Part model, mm, in its own coordinate system. A direction names the side the tool comes from. Coordinates: 2 decimals unless noted, no trailing zeros. Loops run counter-clockwise (first coordinate to the right, second up) from the corner with the lowest first, then second, coordinate; pieces in that order, holes last. Notation, with made-up numbers: (-16.5, -2.5) - (30.5, -2.5) arc R26 cw to (30.5, 17.5) - close; hole circle Ø7 at (-20.5, 66.5). An arc over 180 degrees is marked (long way). Use a Markdown table: item, result. Add a question column.
1) Band-saw the part on C-C (x = 13.5). Give the cut face in (y, z), plus the area to 3 significant figures.
2) Band-saw the part on D-D (z = 18.5). Give the cut face in (x, y).
3) Tool access for faces 5 (the face through (1.5, -2, 30)), 6 (the face through (5.301, -2.465, 5.285)), 7 (the face through (20, -2, -1.5)): list every direction of +Z, -Z, +X, -X, +Y, -Y with a clear straight run to the whole face (end or side of a thin tool).
4) Band-saw the part on B-B (y = -1.7). Give the cut face in (x, z), plus the area to 3 significant figures.
5) Pull direction X, two halves, no side cores. Call faces 1 (the face through (14, -2, 5)), 2 (the face through (-0.54, -2.46, -2.44)), 3 (the face through (-5, -2, 16)), 4 (the face through (4.715, -2.465, 32.699)): +X half, -X half, draft (parallel to the pull), parting line (faces both ways), or undercut.
6) Probe probe 1 along Z at (x, y) = (0, -2.6); probe 2 along X at (y, z) = (-1.5, 27). List the from-to ranges inside material, lowest first. Write a range as [from, to].
7) Band-saw the part on A-A (z = 27.5). Give the cut face in (x, y), plus the area to 3 significant figures.
8) Drop flat-ended pins along their axis: P1, Ø1.5, axis at x = 0.5, z = 27.5, coming from the +Y side; P2, Ø2.5, axis at y = -3, z = 22.5, coming from the +X side. Give the stop position or say it passes through.
from build123d import *

# Parameters (mm, degrees)
F0_R     = 2.5
F1_DEPTH = 5


with BuildPart() as f1:
    # F0 (on Front) → F1 (new body)
    with BuildSketch(Plane.XZ):
        with BuildLine():
            Line((-2.5, 33), (-4, 33))
            ThreePointArc((-4, 33), (-4.707107, 32.707107), (-5, 32))
            Line((-5, 32), (-5, 0))
            ThreePointArc((-5, 0), (-3.535534, -3.535534), (0, -5))
            Line((0, -5), (22.5, -5))
            ThreePointArc((22.5, -5), (23.207107, -4.707107), (23.5, -4))
            Line((23.5, -4), (23.5, -2.5))
            ThreePointArc((23.5, -2.5), (23.207107, -1.792893), (22.5, -1.5))
            Line((22.5, -1.5), (17.5, -1.5))
            ThreePointArc((17.5, -1.5), (16, 0), (17.5, 1.5))
            Line((17.5, 1.5), (22.5, 1.5))
            ThreePointArc((22.5, 1.5), (23.207107, 1.792893), (23.5, 2.5))
            Line((23.5, 2.5), (23.5, 4))
            ThreePointArc((23.5, 4), (23.207107, 4.707107), (22.5, 5))
            Line((22.5, 5), (6, 5))
            ThreePointArc((6, 5), (5.292893, 5.292893), (5, 6))
            Line((5, 6), (5, 32))
            ThreePointArc((5, 32), (4.707107, 32.707107), (4, 33))
            Line((4, 33), (2.5, 33))
            ThreePointArc((2.5, 33), (1.792893, 32.707107), (1.5, 32))
            Line((1.5, 32), (1.5, 27))
            ThreePointArc((1.5, 27), (0, 25.5), (-1.5, 27))
            Line((-1.5, 27), (-1.5, 32))
            ThreePointArc((-1.5, 32), (-1.792893, 32.707107), (-2.5, 33))
        make_face()
        Circle(F0_R, mode=Mode.SUBTRACT)
    extrude(amount=F1_DEPTH)


solid = f1.part
Answer block:
| question | item | result |
|---|---|---|
| 1 | outline | (-5, -5) - (0, -5) - (0, 5) - (-5, 5) - close |
| 1 | area | 50.0 mm2 |
| 2 | outline | (-5, -5) - (5, -5) - (5, 0) - (-5, 0) - close |
| 3 | face 5 | +Z, +Y, -Y |
| 3 | face 6 | +Z, +X, +Y, -Y |
| 3 | face 7 | +X, +Y, -Y |
| 4 | outline | (-5, 0) arc R5 ccw to (0, -5) - (22.5, -5) arc R1 ccw to (23.5, -4) - (23.5, -2.5) arc R1 ccw to (22.5, -1.5) - (17.5, -1.5) arc R1.5 cw to (17.5, 1.5) - (22.5, 1.5) arc R1 ccw to (23.5, 2.5) - (23.5, 4) arc R1 ccw to (22.5, 5) - (6, 5) arc R1 cw to (5, 6) - (5, 32) arc R1 ccw to (4, 33) - (2.5, 33) arc R1 ccw to (1.5, 32) - (1.5, 27) arc R1.5 cw to (-1.5, 27) - (-1.5, 32) arc R1 ccw to (-2.5, 33) - (-4, 33) arc R1 ccw to (-5, 32) - close; hole circle Ø5 at (0, 0) |
| 4 | area | 495 mm2 |
| 5 | face 1 | draft |
| 5 | face 2 | undercut |
| 5 | face 3 | -X half |
| 5 | face 4 | +X half |
| 6 | probe 1 | [-5, -2.5], [2.5, 25.5] |
| 6 | probe 2 | [-5, -1.5], [1.5, 5] |
| 7 | outline | (-5, -5) - (-1.5, -5) - (-1.5, 0) - (-5, 0) - close; (1.5, -5) - (5, -5) - (5, 0) - (1.5, 0) - close |
| 7 | area | 35.0 mm2 |
| 8 | P1 | through |
| 8 | P2 | x = 5 |
